Work out the finished part from the listing and answer in its coordinate system (mm). A direction names the side the tool comes from. Give positions to 0.01 mm unless a question says otherwise; leave off trailing zeros. Order: outer loops, then holes, each group sorted by start corner. A loop starts at its lowest first (then second) coordinate and runs counter-clockwise, first axis right, second up. Notation, with made-up numbers: (36.5, 63.25) - (83.5, 63.25) arc R13 ccw to (83.5, 78.25) - close; hole circle Ø2 at (63.5, 61.5). An arc over 180 degrees is marked (long way). Write each question's results on one line, items separated by ' | '.
from build123d import *

# Parameters (mm, degrees)
SKETCH1_R           = 1
BOSS_EXTRUDE1_DEPTH = 11
FILLET1_R           = 5
FILLET2_R           = 1


with BuildPart() as part:
    # Sketch1 → Boss-Extrude1 (new body, symmetric)
    with BuildSketch(Plane.XY):
        Polygon((35.5, -13), (-11.5, -13), (-11.5, 13), (35.5, 13), (35.5, 5.75), (37, 5.75), (37, -5.75), (35.5, -5.75), align=None)
        with Locations((-9, 9.25)):
            Circle(SKETCH1_R, mode=Mode.SUBTRACT)
        with Locations((33, 10.4)):
            Circle(SKETCH1_R, mode=Mode.SUBTRACT)
        with Locations((33, -10.4)):
            Circle(SKETCH1_R, mode=Mode.SUBTRACT)
        with Locations((-9, -9.25)):
            Circle(SKETCH1_R, mode=Mode.SUBTRACT)
    extrude(amount=BOSS_EXTRUDE1_DEPTH, both=True)

    # Fillet1
    fillet1_edges = [part.edges().sort_by_distance(p)[0] for p in [
        (-11.5, 13, 0),
        (-11.5, -13, 0),
    ]]
    fillet(fillet1_edges, radius=FILLET1_R)

    # Fillet2
    fillet2_edges = [part.edges().sort_by_distance(p)[0] for p in [
        (35.5, 13, 0),
        (35.5, -13, 0),
    ]]
    fillet(fillet2_edges, radius=FILLET2_R)


solid = part.part
1. A cutting plane is placed at C-C, the plane x = -9. Write down the section's boundary in (y, z), then the cut area to 3 significant figures.
Answer list:
outline: (-12.33, -11) - (-10.25, -11) - (-10.25, 11) - (-12.33, 11) - close; (-8.25, -11) - (8.25, -11) - (8.25, 11) - (-8.25, 11) - close; (10.25, -11) - (12.33, -11) - (12.33, 11) - (10.25, 11) - close | area: 455 mm^2
2. Given P1, Ø1.2, axis at x = 33, y = -10.4, coming from the +Z side; P2, Ø1.9, axis at y = -9.5, z = 5, coming from the +X side, each flat-ended and moving along its own axis, determine where each tip first touches the part or whether it passes through.
Answer list:
P1: through | P2: x = 35.5
3. A cutting plane is placed at B-B, the plane z = -1.75. Write down the section's boundary in (x, y).
Answer list:
outline: (-11.5, -8) arc R5 ccw to (-6.5, -13) - (34.5, -13) arc R1 ccw to (35.5, -12) - (35.5, -5.75) - (37, -5.75) - (37, 5.75) - (35.5, 5.75) - (35.5, 12) arc R1 ccw to (34.5, 13) - (-6.5, 13) arc R5 ccw to (-11.5, 8) - close; hole circle Ø2 at (-9, -9.25); hole circle Ø2 at (-9, 9.25); hole circle Ø2 at (33, -10.4); hole circle Ø2 at (33, 10.4)
4. A tool of negligible diameter and unlimited length cuts with its end or side. For faces 1 (the face through (36, 5.75, 0)), 2 (the face through (13, 0, 11)), 3 (the face through (36, -5.75, 0)), from which of +Z, -Z, +X, -X, +Y, -Y can it reach the whole face along a straight path? Write none if from no direction.
Answer list:
face 1: +Z, -Z, +X, +Y | face 2: +Z, +X, -X, +Y, -Y | face 3: +Z, -Z, +X, -Y
5. Straight lines are drawn through the part: line 1 (Y direction, x = 33, z = 5.5); line 2 (Y direction, x = -9, z = 4); line 3 (X direction, y = -11, z = -1). For each, find the intervals that lie inside material, in ascending order. Write a range as [from, to].
Answer list:
line 1: [-13, -11.4], [-9.4, 9.4], [11.4, 13] | line 2: [-12.33, -10.25], [-8.25, 8.25], [10.25, 12.33] | line 3: [-10.5, 32.2], [33.8, 35.5]
6. A cutting plane is placed at A-A, the plane x = 33. Write down the section's boundary in (y, z).
Answer list:
outline: (-13, -11) - (-11.4, -11) - (-11.4, 11) - (-13, 11) - close; (-9.4, -11) - (9.4, -11) - (9.4, 11) - (-9.4, 11) - close; (11.4, -11) - (13, -11) - (13, 11) - (11.4, 11) - close
7. A cutting plane is placed at D-D, the plane y = -6.75. Write down the section's boundary in (x, z).
Answer list:
outline: (-11.5, -11) - (35.5, -11) - (35.5, 11) - (-11.5, 11) - close
8. Determine the mould class of faces 4 (the face through (-9.13, 10.24, -0.15)), 5 (the face through (-9.13, -8.26, -0.15)), 6 (the face through (35.5, 9, 0)), 7 (the face through (-10, 11.57, -0.15)) for opening direction Y: +Y half, -Y half, draft (parallel to the pull), parting line (faces both ways), or undercut.
Answer list:
face 4: undercut | face 5: undercut | face 6: draft | face 7: +Y half
